Here's the drawing with two shaded views (mm, measured from the low corner). I have some questions. Coordinates: 2 decimals unless noted, no trailing zeros. Write each loop counter-clockwise with the first axis right and the second up, starting at its lowest first coordinate (ties: lowest second). Pieces come first, ordered by that corner, then holes. Notation, with made-up numbers: (0, 89.5) -> (52, 89.5) arc R15 cw to (52, 98.5) -> close; hole circle Ø10 at (10.25, 62). An arc over 180 degrees is marked (long way). Answer in a Markdown table with one row per item. Add a question column.
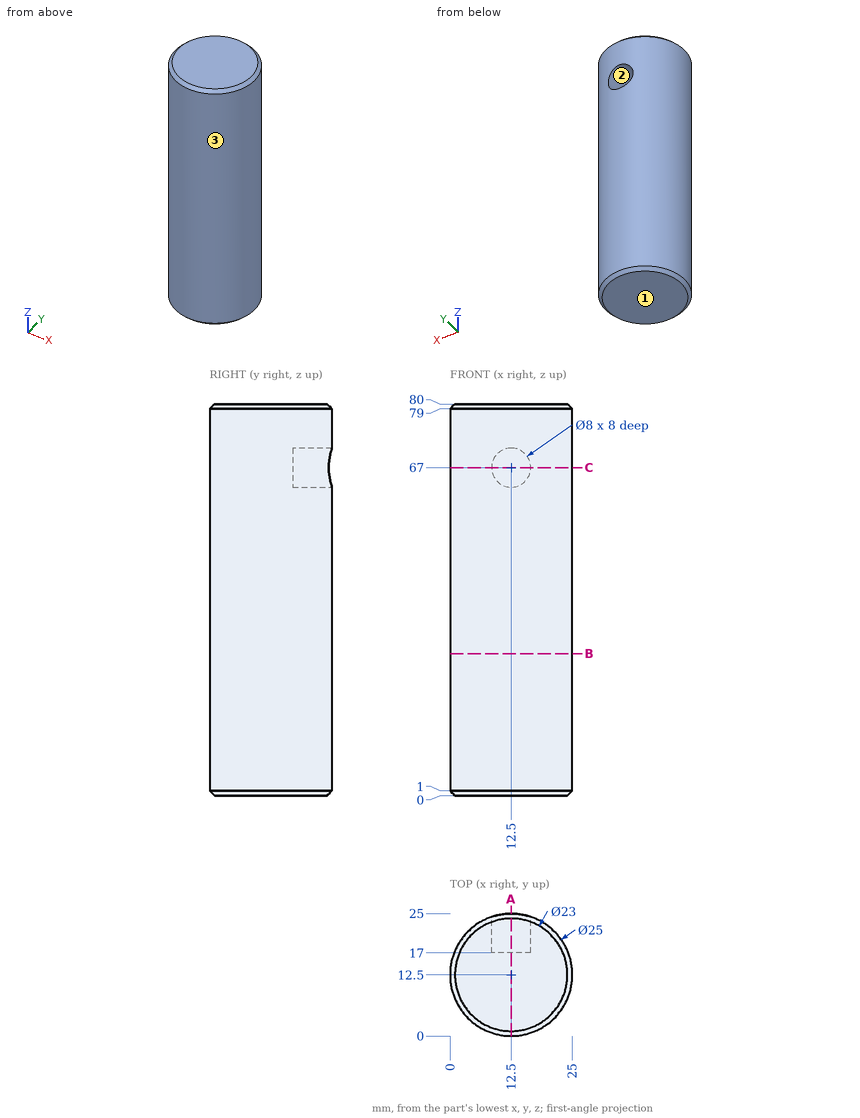
Q1. Imagine slicing it at A-A on x = 12.5. Please give me the cut outline in (y, z), plus the area to 3 significant figures.
Q2. I need wall thicknesses on line 1 (X direction, y = 18.75, z = 67); line 2 (X direction, y = 22, z = 67); line 3 (X direction, y = 13, z = 73). Which ranges of each line are inside material? Lowest first, please. Write a range as [from, to].
Q3. Imagine slicing it at B-B on z = 29. Please give me the cut outline in (x, y), plus the area to 3 significant figures.
Q4. Imagine slicing it at C-C on z = 67. Please give me the cut outline in (x, y), plus the area to 3 significant figures.
Q5. If we mould it in two halves opening along X, with no side actions, what happens to the marked faces 1, 2 and 3? For each: pulls with the +X half, pulls with the -X half, needs draft (parallel to the pull), parting line crosses it, or undercut.
Q6. I'm going to push flat-ended pins straight in: P1, Ø8, axis at x = 22, z = 68, coming from the +Y side (3 decimals); P2, Ø1, axis at y = 22, z = 50, coming from the -X side; P3, Ø7, axis at x = 12.5, z = 67, coming from the +Y side. Where does each tip first touch, or does it pass through?
Result sheet:
| question | item | result |
|---|---|---|
| 1 | outline | (0, 1) -> (1, 0) -> (24, 0) -> (25, 1) -> (25, 63) -> (17, 63) -> (17, 71) -> (25, 71) -> (25, 79) -> (24, 80) -> (1, 80) -> (0, 79) -> close |
| 1 | area | 1,930 mm^2 |
| 2 | line 1 | x = [1.67, 8.5], [16.5, 23.33] |
| 2 | line 2 | x = [4.38, 8.5], [16.5, 20.62] |
| 2 | line 3 | x = [0.01, 24.99] |
| 3 | outline | circle Ø25 at (12.5, 12.5) |
| 3 | area | 491 mm^2 |
| 4 | outline | (8.5, 17) -> (8.5, 24.34) arc R12.5 ccw (long way) to (16.5, 24.34) -> (16.5, 17) -> close |
| 4 | area | 429 mm^2 |
| 5 | face 1 | needs draft |
| 5 | face 2 | undercut |
| 5 | face 3 | parting line crosses it |
| 6 | P1 | stops at y = 23.725 |
| 6 | P2 | stops at x = 3.83 |
| 6 | P3 | stops at y = 17 |
